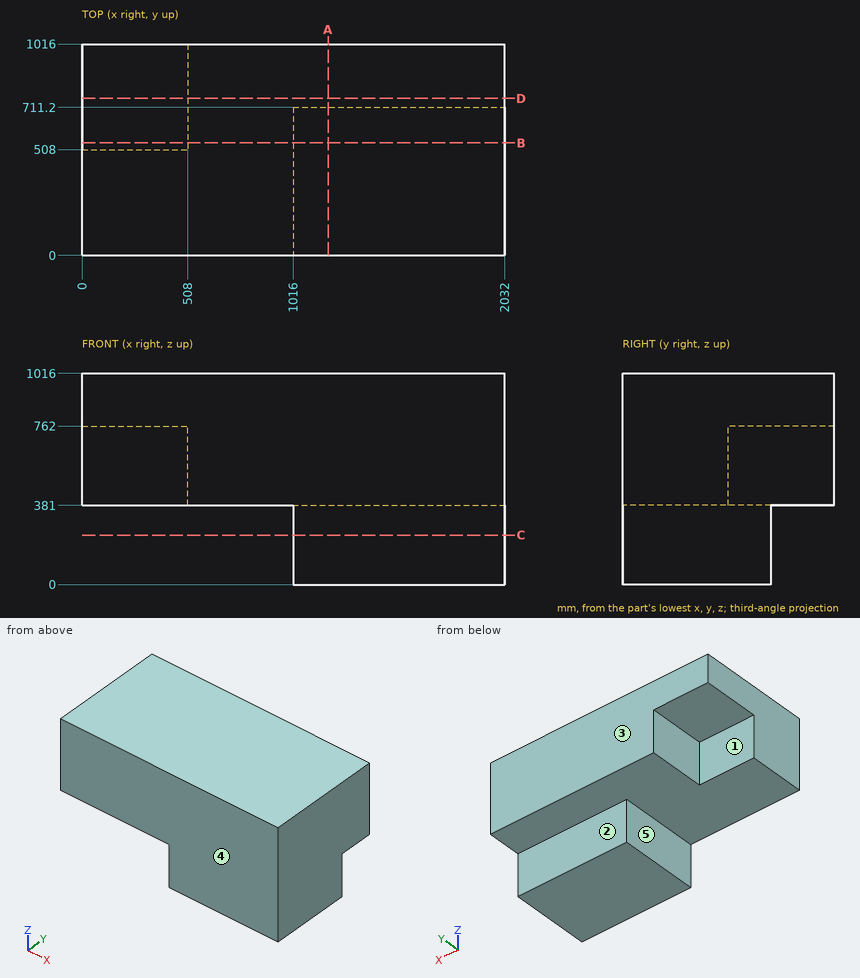
Check sheet for the drawn part. Datum: minimum x, y, z corner. Units: mm. A direction names the side the tool comes from. Round coordinates to 2 decimals unless told otherwise and drop trailing zeros. Order: outer loops, then holes, each group sorted by start corner. A loop starts at its lowest first (then second) coordinate and runs counter-clockwise, first axis right, second up.
1) Go/stop test with flat-tipped pins: pin 1 Ø2 at (y, z) = (444.5, 316) entering from -X; pin 2 Ø4 at (x, y) = (218.5, 592.5) entering from -Z. Record where each tip stops, or that it passes through.
2) Section check B-B (y = 540.5). Record the boundary of the cut face in (x, z), and give its area (3 significant figures).
3) Section check C-C (z = 238). Record the boundary of the cut face in (x, y), and give its area (3 significant figures).
4) Scan lines: line 1 (Z direction, x = 747, y = 253.5); line 2 (X direction, y = 563, z = 681); line 3 (X direction, y = 403.5, z = 111.5). Record each from-to range of solid material in increasing order.
5) Section check D-D (y = 754.5). Record the boundary of the cut face in (x, z).
6) Section check A-A (x = 1183.5). Record the boundary of the cut face in (y, z), and give its area (3 significant figures).
7) Tool access check on the marked faces 1, 2, 3, 4 and 5. Record the directions out of +Z, -Z, +X, -X, +Y, -Y that give a thin tool (end or side, any length) a straight path to the whole face; none if there is none.
Result:
1. pin 1: stops at x = 1016
1. pin 2: stops at z = 762
2. outline: (0, 762) - (508, 762) - (508, 381) - (1016, 381) - (1016, 0) - (2032, 0) - (2032, 1016) - (0, 1016) - close
2. area: 1,480,000 mm2
3. outline: (1016, 0) - (2032, 0) - (2032, 711.2) - (1016, 711.2) - close
3. area: 723,000 mm2
4. line 1: z = 381 to 1016
4. line 2: x = 508 to 2032
4. line 3: x = 1016 to 2032
5. outline: (0, 762) - (508, 762) - (508, 381) - (2032, 381) - (2032, 1016) - (0, 1016) - close
6. outline: (0, 0) - (711.2, 0) - (711.2, 381) - (1016, 381) - (1016, 1016) - (0, 1016) - close
6. area: 916,000 mm2
7. face 1: -Z, -X, +Y
7. face 2: -Z, +X, -X, +Y
7. face 3: +Z, -Z, +X, -X, +Y
7. face 4: +Z, -Z, +X, -X, -Y
7. face 5: -Z, -X, +Y, -Y
